Part model, mm, in its own coordinate system. A direction names the side the tool comes from. Coordinates: 2 decimals unless noted, no trailing zeros. Order: outer loops, then holes, each group sorted by start corner. A loop starts at its lowest first (then second) coordinate and runs counter-clockwise, first axis right, second up.
from build123d import *

# Parameters (mm, degrees)
SKETCH1_R           = 50
BOSS_EXTRUDE1_DEPTH = 15
SKETCH6_R           = 32.5
BOSS_EXTRUDE2_DEPTH = 35
SKETCH7_R           = 32.5
BOSS_EXTRUDE3_DEPTH = 3
BOSS_EXTRUDE3_TAPER = 60
SKETCH9_R           = 25.75
CUT_EXTRUDE5_DEPTH  = 10.2
SKETCH10_R          = 20
CUT_EXTRUDE6_DEPTH  = 83.654945457
SKETCH11_R          = 4.05
CUT_EXTRUDE7_DEPTH  = 40
CIRPATTERN1_COUNT   = 4
CHAMFER1_SIZE       = 3


with BuildPart() as part:
    # Sketch1 → Boss-Extrude1 (new body)
    with BuildSketch(Plane.XZ.offset(-11.5)):
        with Locations(Location((0, 0, 0), (0, 0, 90))):
            Circle(SKETCH1_R)
    extrude(amount=-BOSS_EXTRUDE1_DEPTH)

    # Sketch6 → Boss-Extrude2 (add)
    with BuildSketch(Plane(origin=(0, 26.5, 0), x_dir=(-1, 0, 0), z_dir=(0, 1, 0))):
        with Locations(Location((0, 0, 0), (0, 0, 90))):
            Circle(SKETCH6_R)
    extrude(amount=BOSS_EXTRUDE2_DEPTH)

    # Sketch7 → Boss-Extrude3 (add)
    with BuildSketch(Plane(origin=(0, 61.5, 0), x_dir=(-1, 0, 0), z_dir=(0, 1, 0))):
        with Locations(Location((0, 0, 0), (0, 0, 90))):
            Circle(SKETCH7_R)
    extrude(amount=BOSS_EXTRUDE3_DEPTH, taper=BOSS_EXTRUDE3_TAPER)

    # Sketch9 → Cut-Extrude5 (cut)
    with BuildSketch(Plane.XZ.offset(-11.5)):
        with Locations(Location((0, 0, 0), (0, 0, 90))):
            Circle(SKETCH9_R)
    extrude(amount=-CUT_EXTRUDE5_DEPTH, mode=Mode.SUBTRACT)

    # Sketch10 → Cut-Extrude6 (cut, through all)
    with BuildSketch(Plane.XZ.offset(-21.7)):
        with Locations(Location((0, 0, 0), (0, 0, 90))):
            Circle(SKETCH10_R)
    extrude(amount=-CUT_EXTRUDE6_DEPTH, mode=Mode.SUBTRACT)

    # Sketch11 → Cut-Extrude7 (cut)
    with BuildSketch(Plane(origin=(389.160069558, 11.5, 0), x_dir=(1, 0, 0), z_dir=(0, 1, 0))):
        with Locations(Location((-360.168691529, 28.991378029, 0), (0, 0, 270))):
            Circle(SKETCH11_R)
    cut_extrude7 = extrude(amount=CUT_EXTRUDE7_DEPTH, mode=Mode.SUBTRACT)

    # CirPattern1: Cut-Extrude7 ×4 about axis
    cirpattern1_axis = Axis((0, 0, 0), (0, 1, 0))
    for i in range(1, CIRPATTERN1_COUNT):
        add(cut_extrude7.rotate(cirpattern1_axis, i * 360 / CIRPATTERN1_COUNT), mode=Mode.SUBTRACT)

    # Chamfer1
    chamfer1_edges = [part.edges().sort_by_distance(p)[0] for p in [
        (0, 26.5, -50),
    ]]
    chamfer(chamfer1_edges, length=CHAMFER1_SIZE)


solid = part.part
Q1. Cut at C-C on y = 46. Write the cut outline in (x, z).
Results list:
outline: circle Ø65 at (0, 0); hole circle Ø40 at (0, 0)
Q2. Wall check: line 1 along Z through (x, y) = (-0.5, 36); line 2 along X through (y, z) = (50, 0); line 3 along Y through (x, z) = (10.5, 42). Give the ranges that are in metal, low to high.
Results list:
line 1: z = -32.5 to -19.99, 19.99 to 32.5
line 2: x = -32.5 to -20, 20 to 32.5
line 3: y = 11.5 to 26.5
Q3. Cut at A-A on z = 0. Write the cut outline in (x, y).
Results list:
outline: (-50, 11.5) - (-25.75, 11.5) - (-25.75, 21.7) - (-20, 21.7) - (-20, 64.5) - (-27.3, 64.5) - (-32.5, 61.5) - (-32.5, 26.5) - (-47, 26.5) - (-50, 23.5) - close; (20, 21.7) - (25.75, 21.7) - (25.75, 11.5) - (50, 11.5) - (50, 23.5) - (47, 26.5) - (32.5, 26.5) - (32.5, 61.5) - (27.3, 64.5) - (20, 64.5) - close
Q4. Cut at B-B on y = 18. Write the cut outline in (x, z).
Results list:
outline: circle Ø100 at (0, 0); hole circle Ø8.1 at (-28.99, -28.99); hole circle Ø8.1 at (-28.99, 28.99); hole circle Ø51.5 at (0, 0); hole circle Ø8.1 at (28.99, -28.99); hole circle Ø8.1 at (28.99, 28.99)
Q5. Pin check, flat tips, straight feed: pin 1 Ø1 at (y, z) = (34, -14.5) entering from -X; pin 2 Ø3 at (x, y) = (31, 49.5) entering from +Z; pin 3 Ø5 at (x, z) = (-2.5, -37.5) entering from +Y; pin 4 Ø13 at (x, z) = (28.99, 28.99) entering from -Y. Stop position of each tip, or through.
Results list:
pin 1: stops at x = -29.33
pin 2: stops at z = 13.64
pin 3: stops at y = 26.5
pin 4: stops at y = 11.5
Q6. Which spindle directions (+Z, -Z, +X, -X, +Y, -Y) get a long thin tool onto all of the face, cutting with end or side? Do faces 4 (the face through (22.845, 16.529, 11.882)), 5 (the face through (32.21, 18.9, 26.53)). Say none if no direction does.
Results list:
face 4: -Y
face 5: +Y, -Y
Q7. Cut at D-D on z = 30.5. Count the separate pieces of the cut face and the enclosed holes in it, and give its area (3 significant figures).
Results list:
separate pieces: 3
enclosed holes: 0
area: 1,750 mm2
Q8. Mould opens along X. For faces 1 (the face through (9.76, 43.76, 31)), 2 (the face through (31, 26.5, -11)), 3 (the face through (13.2, 21.7, -15.4)) say: pulls with the +X half, pulls with the -X half, needs draft (parallel to the pull), parting line crosses it, or undercut.
Results list:
face 1: parting line crosses it
face 2: needs draft
face 3: undercut
